```python
from build123d import *

# Parameters (mm, degrees)
F0_W          = 2.54
F0_H          = 12.7
F3_DEPTH      = 25.4
F2_R          = 69.85
F4_DEPTH      = 25.4
F4_DEPTH_BACK = 25.4


with BuildPart() as f1:
    # F0 (on Front) → F1 (revolve)
    with BuildSketch(Plane.XZ):
        with Locations((-6.0325, 6.35)):
            Rectangle(F0_W, F0_H)
        Polygon((-7.3025, 12.7), (-4.7625, 12.7), (-4.7625, 15.24), (-11.1125, 15.24), (-11.1125, 12.7), align=None)
    revolve(axis=Axis((0, 0, 2.0128042901), (0, 0, 1)))

    # F3 (add): a face of the model
    f3_faces = [f1.faces().sort_by_distance(p)[0] for p in [
        (7.0959541092, 0, 0),
    ]]
    extrude(f3_faces, amount=F3_DEPTH)

    # F2 (on Front) → F4 (cut, two sides)
    with BuildSketch(Plane.XZ) as f4_sk:
        with Locations((0, -69.85)):
            Circle(F2_R)
    extrude(amount=-F4_DEPTH, mode=Mode.SUBTRACT)
    extrude(f4_sk.sketch, amount=F4_DEPTH_BACK, mode=Mode.SUBTRACT)


solid = f1.part
```
Model file for the job. Use its own axes, mm. A direction names the side the tool comes from. Round coordinates to 2 decimals unless told otherwise and drop trailing zeros. Write each loop counter-clockwise with the first axis right and the second up, starting at its lowest first coordinate (ties: lowest second). Pieces come first, ordered by that corner, then holes. Notation, with made-up numbers: M 29,-15.5 L 86,-15.5 A16 ccw 86,4.5 Z; hole C 24.25,37.25 d9. An arc over 180 degrees is marked long. Put each result on its own line as item: value.
Item 1: Cut at D-D (x = -6.75). List the corners of the cut face in (y, z), and give its area (3 significant figures).
Responses:
outline: M -8.83,12.7 L -2.79,12.7 L -2.79,-0.33 L 2.79,-0.33 L 2.79,12.7 L 8.83,12.7 L 8.83,15.24 L -8.83,15.24 Z
area: 117 mm²
Item 2: Cut at C-C (z = 4). List the corners of the cut face in (x, y) (1 decimal).
Responses:
outline: C 0,0 d14.6; hole C 0,0 d9.5
Item 3: Cut at B-B (y = -3.25). List the corners of the cut face in (x, z).
Responses:
outline: M -10.63,12.7 L -6.54,12.7 L -6.54,-0.31 A69.85 cw -3.48,-0.09 L -3.48,15.24 L -10.63,15.24 Z; M 3.48,-0.09 A69.85 cw 6.54,-0.31 L 6.54,12.7 L 10.63,12.7 L 10.63,15.24 L 3.48,15.24 Z
Item 4: Flat gauge pins, fed straight in: P1, Ø6, axis at x = 0.5, z = 5, coming from the +Y side; P2, Ø6, axis at x = -6.5, z = 6, coming from the -Y side; P3, Ø8, axis at x = 1.5, z = 8.5, coming from the -Y side. Where does each tip first touch, or does it go through?
Responses:
P1: y = 7.3
P2: y = -6.41
P3: y = -7.3
Item 5: Tool access for faces 1 (the cylindrical face through (0, 5, 0)), 2 (the cylindrical face through (5.38, -4.94, 6.25)): list every direction of +Z, -Z, +X, -X, +Y, -Y with a clear straight run to the whole face (end or side of a thin tool).
Responses:
face 1: -Z, +Y, -Y
face 2: -Z
Item 6: Probe L1, parallel to Y at x = 0, z = 10.75; L2, parallel to Z at x = 7.25, y = 0. List the from-to ranges inside material, lowest first. Write a range as from..to.
Responses:
L1: -7.3..-4.76, 4.76..7.3
L2: -0.38..15.24
Item 7: Cut at A-A (x = 0). List the corners of the cut face in (y, z), and give its area (3 significant figures).
Responses:
outline: M -11.11,12.7 L -7.3,12.7 L -7.3,0 L -4.76,0 L -4.76,15.24 L -11.11,15.24 Z; M 4.76,0 L 7.3,0 L 7.3,12.7 L 11.11,12.7 L 11.11,15.24 L 4.76,15.24 Z
area: 96.8 mm²
